Model file for the job. Use its own axes, mm. Give positions to 0.01 mm unless a question says otherwise; leave off trailing zeros. Write each loop counter-clockwise with the first axis right and the second up, starting at its lowest first coordinate (ties: lowest second). Pieces come first, ordered by that corner, then holes. Notation, with made-up numbers: (64.25, 74) - (112.25, 74) arc R29 cw to (112.25, 105) - close; hole circle Ø1 at (39.5, 89). An arc over 180 degrees is marked (long way). Use a Markdown table: item, result. Add a question column.
```python
from build123d import *

# Parameters (mm, degrees)
SKETCH1_R           = 20
BOSS_EXTRUDE1_DEPTH = 20
SKETCH2_R           = 20
SKETCH3_R           = 1
CUT_EXTRUDE1_DEPTH  = 35.641016151


with BuildPart() as part:
    # Sketch1 → Boss-Extrude1 (new body)
    with BuildSketch(Plane(origin=(0, 0, 0), x_dir=(1, 0, 0), z_dir=(0, 1, 0))):
        with Locations(Location((0, 0, 0), (0, 0, 270))):
            Circle(SKETCH1_R)
    extrude(amount=BOSS_EXTRUDE1_DEPTH)

    # Sketch2 → Cut-Revolve1 (revolve, cut)
    with BuildSketch(Plane(origin=(0, 0, 0), x_dir=(0, 0, -1), z_dir=(1, 0, 0))):
        with Locations((37.320508076, 10)):
            Circle(SKETCH2_R)
    revolve(axis=Axis((0, 0, 0), (0, 1, 0)), mode=Mode.SUBTRACT)

    # Sketch3 → Cut-Extrude1 (cut, through all)
    with BuildSketch(Plane(origin=(0, 20, 0), x_dir=(1, 0, 0), z_dir=(0, 1, 0))):
        with Locations(Location((0, 0, 0), (0, 0, 270))):
            Circle(SKETCH3_R)
    extrude(amount=-CUT_EXTRUDE1_DEPTH, mode=Mode.SUBTRACT)


solid = part.part
```
(1) Band-saw the part on B-B (x = 0). Write the cut outline in (y, z), then the cut area to 3 significant figures.
(2) Flat gauge pins, fed straight in: pin 1 (1 mm diameter, centred on x = 2.5, y = 17.5, fed in from +Z); pin 2 (8 mm diameter, centred on y = 3.5, z = -2.5, fed in from +X); pin 3 (1.5 mm diameter, centred on y = 15, z = -15.5, fed in from +X). Where does each tip first touch, or does it go through?
(3) Band-saw the part on C-C (y = 5.25). Write the cut outline in (x, z), then the cut area to 3 significant figures.
(4) Probe probe 1 along X at (y, z) = (4.5, 0); probe 2 along X at (y, z) = (1.5, -8); probe 3 along Z at (x, y) = (-8, 15.5). List the from-to ranges inside material, lowest first. Write a range as [from, to].
(5) Band-saw the part on D-D (y = 13.75). Write the cut outline in (x, z).
(6) Band-saw the part on A-A (z = 0). Write the cut outline in (x, y).
(7) Two-plate mould, pull along X, no slides. Class faces 1 (the flat face through (0, 20, 4)), 2 (the cylindrical face through (-1, 10, 0)): +X half, -X half, draft (parallel to the pull), parting line (faces both ways), or undercut.
Model answer:
| question | item | result |
|---|---|---|
| 1 | outline | (0, -20) arc R20 cw to (20, -20) - (20, -1) - (0, -1) - close; (0, 1) - (20, 1) - (20, 20) arc R20 cw to (0, 20) - close |
| 1 | area | 688 mm^2 |
| 2 | pin 1 | stops at z = 18.83 |
| 2 | pin 2 | stops at x = 19.99 |
| 2 | pin 3 | stops at x = 10.29 |
| 3 | outline | circle Ø35.79 at (0, 0); hole circle Ø2 at (0, 0) |
| 3 | area | 1,000 mm^2 |
| 4 | probe 1 | x = [-18.09, -1], [1, 18.09] |
| 4 | probe 2 | x = [-17.47, 17.47] |
| 4 | probe 3 | z = [-16.23, 16.23] |
| 5 | outline | circle Ø35.35 at (0, 0); hole circle Ø2 at (0, 0) |
| 6 | outline | (-20, 0) - (-1, 0) - (-1, 20) - (-20, 20) arc R20 cw to start; (1, 0) - (20, 0) arc R20 cw to (20, 20) - (1, 20) - close |
| 7 | face 1 | draft |
| 7 | face 2 | undercut |
